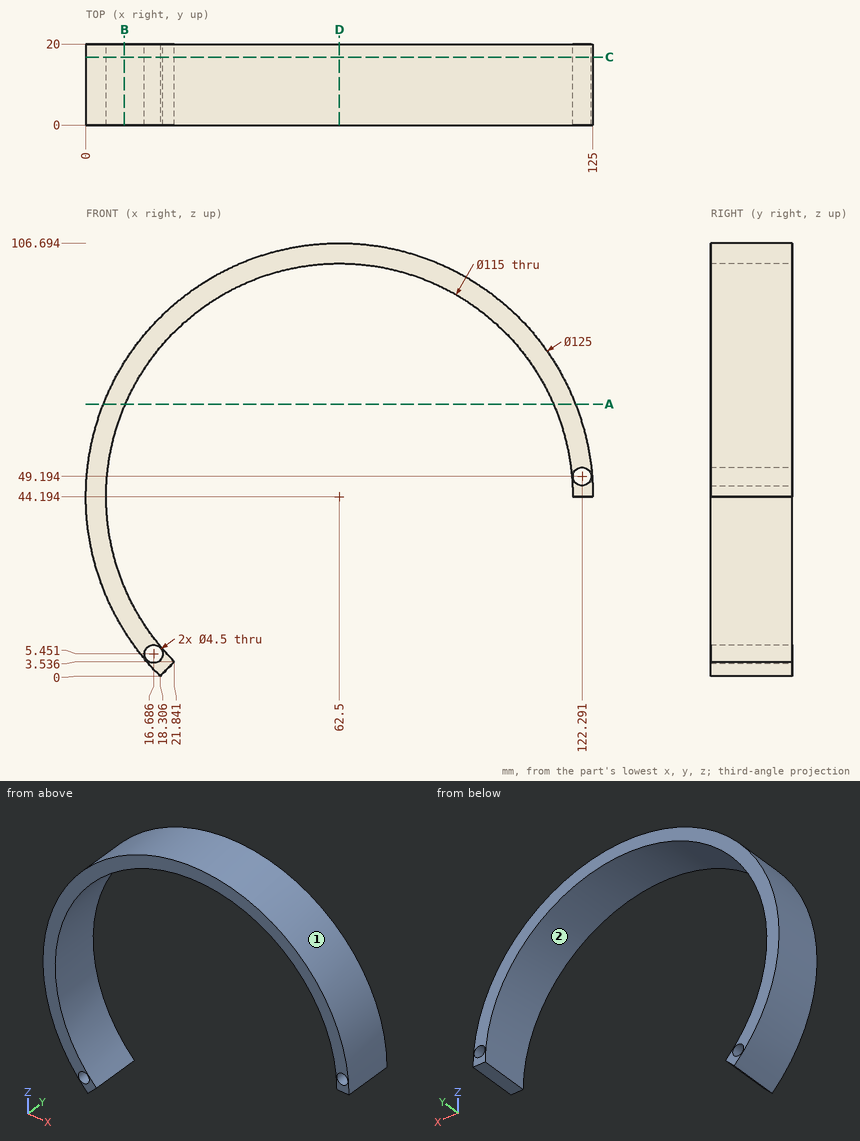
Study the drawing (mm; zero at the part's minimum x, y, z) and answer. Coordinates: 2 decimals unless noted, no trailing zeros. Write each loop counter-clockwise with the first axis right and the second up, starting at its lowest first coordinate (ties: lowest second). Pieces come first, ordered by that corner, then holes. Notation, with made-up numbers: M 15.5,4 L 42.5,4 A14 cw 42.5,28 Z; hole C 68,6.25 d9. An arc over 180 degrees is marked long. Write each question's results on one line, items separated by ' | '.
Item 1: For a pull along X with two mould halves and no side action, classify the marked faces 1 and 2 as released by +X, released by -X, zero draft, split by the parting line, or undercut.
Answer below:
face 1: split by the parting line | face 2: undercut
Item 2: The part is cut by section D-D on x = 62.5. Determine the outline of the cut face in (y, z) (1 decimal).
Answer below:
outline: M 0,101.7 L 20,101.7 L 20,106.7 L 0,106.7 Z
Item 3: The part is cut by section C-C on y = 16.75. State how many separate pieces and enclosed holes the cut face has, and give its area (3 significant figures).
Answer below:
separate pieces: 1 | enclosed holes: 2 | area: 1,150 mm2
Item 4: Consider probe 1 along Z at (x, y) = (15, 3.75) (1 decimal); probe 2 along X at (y, z) = (11.25, 46); probe 3 along Z at (x, y) = (62.5, 7.5) (1 decimal). Determine where each line is inside the solid, lowest interval first. Write a range as [from, to].
Answer below:
probe 1: [3.6, 4], [6.9, 11.8], [76.6, 84.8] | probe 2: [0.03, 5.03], [119.97, 124.97] | probe 3: [101.7, 106.7]
Item 5: Given P1, Ø4, axis at x = 55, y = 14.5, coming from the -Z side; P2, Ø10, axis at x = 48.5, y = 11, coming from the +Z side; P3, Ø4, axis at x = 16.69, z = 5.45, coming from the -Y side; P4, Ø1.5, axis at x = 39, y = 5.5, coming from the +Z side, each flat-ended and moving along its own axis, determine where each tip first touches the part or whether it passes through.
Answer below:
P1: z = 100.9 | P2: z = 106.04 | P3: through | P4: z = 102.41
Item 6: The part is cut by section B-B on x = 9.5. Determine the outline of the cut face in (y, z) (1 decimal).
Answer below:
outline: M 0,11.1 L 20,11.1 L 20,21.9 L 0,21.9 Z; M 0,66.5 L 20,66.5 L 20,77.3 L 0,77.3 Z
Item 7: The part is cut by section A-A on z = 67. Determine the outline of the cut face in (x, y), and give its area (3 significant figures).
Answer below:
outline: M 4.31,0 L 9.72,0 L 9.72,20 L 4.31,20 Z; M 115.28,0 L 120.69,0 L 120.69,20 L 115.28,20 Z | area: 216 mm2
